Part model, mm, in its own coordinate system. A direction names the side the tool comes from. Give positions to 0.01 mm unless a question says otherwise; leave off trailing zeros. Order: outer loops, then holes, each group sorted by start corner. A loop starts at its lowest first (then second) coordinate and runs counter-clockwise, first axis right, second up.
1. Slice it at C-C on y = 4.2. List the corners of the cut face in (x, z).
2. Mould opens along X. For faces 1 (the flat face through (0, 2, -27)), 2 (the flat face through (31, 4, 0)), 3 (the cylindrical face through (32.287, 2.535, 26.248)) say: +X half, -X half, draft (parallel to the pull), parting line (faces both ways), or undercut.
3. Drop flat-ended pins along their axis: pin 1 Ø3 at (x, z) = (27, -22.5) entering from +Y; pin 2 Ø25 at (x, z) = (-1.5, 5.5) entering from +Y; pin 3 Ø3 at (x, z) = (-22, -16.5) entering from -Y. Give the stop position or say it passes through.
4. Slice it at B-B on x = -27. List the corners of the cut face in (y, z), and give its area (3 significant figures).
5. Slice it at D-D on z = 12. List the corners of the cut face in (x, y).
6. Slice it at A-A on z = -22. List the corners of the cut face in (x, y).
7. Probe line 1 (X direction, y = 1.1, z = -22); line 2 (Z direction, x = 27, y = 1.7); line 3 (X direction, y = 2.8, z = -22). List the from-to ranges inside material, lowest first.
8. Which spindle directions (+Z, -Z, +X, -X, +Y, -Y) get a long thin tool onto all of the face, cutting with end or side? Do faces 4 (the flat face through (0, 4, -25)), 5 (the cylindrical face through (-28.11, 1.52, -23.01)). Say none if no direction does.
from build123d import *

# Parameters (mm, degrees)
SKETCH1_W           = 66
SKETCH1_H           = 54
BOSS_EXTRUDE1_DEPTH = 5
SKETCH2_W           = 62
SKETCH2_H           = 50
CUT_EXTRUDE1_DEPTH  = 3
SKETCH3_W           = 8
SKETCH3_H           = 6
SKETCH3_R           = 1.5
BOSS_EXTRUDE2_DEPTH = 3
SKETCH4_R           = 1.5
CUT_EXTRUDE2_DEPTH  = 3
FILLET1_R           = 2.5


with BuildPart() as part:
    # Sketch1 → Boss-Extrude1 (new body)
    with BuildSketch(Plane(origin=(0, 0, 0), x_dir=(1, 0, 0), z_dir=(0, 1, 0))):
        Rectangle(SKETCH1_W, SKETCH1_H)
    extrude(amount=BOSS_EXTRUDE1_DEPTH)

    # Sketch2 → Cut-Extrude1 (cut)
    with BuildSketch(Plane(origin=(0, 5, 0), x_dir=(1, 0, 0), z_dir=(0, 1, 0))):
        Rectangle(SKETCH2_W, SKETCH2_H)
    extrude(amount=-CUT_EXTRUDE1_DEPTH, mode=Mode.SUBTRACT)

    # Sketch3 → Boss-Extrude2 (add)
    with BuildSketch(Plane(origin=(0, 0, 0), x_dir=(1, 0, 0), z_dir=(0, 1, 0))):
        with Locations((-27, -22)):
            Rectangle(SKETCH3_W, SKETCH3_H)
        with Locations((-27, -22)):
            Circle(SKETCH3_R, mode=Mode.SUBTRACT)
        with Locations((-27, 22)):
            Rectangle(SKETCH3_W, SKETCH3_H)
        with Locations((-27, 22)):
            Circle(SKETCH3_R, mode=Mode.SUBTRACT)
        with Locations((27, -22)):
            Rectangle(SKETCH3_W, SKETCH3_H)
        with Locations((27, -22)):
            Circle(SKETCH3_R, mode=Mode.SUBTRACT)
        with Locations((27, 22)):
            Rectangle(SKETCH3_W, SKETCH3_H)
        with Locations((27, 22)):
            Circle(SKETCH3_R, mode=Mode.SUBTRACT)
    extrude(amount=BOSS_EXTRUDE2_DEPTH)

    # Sketch4 → Cut-Extrude2 (cut)
    with BuildSketch(Plane(origin=(0, 2, 0), x_dir=(1, 0, 0), z_dir=(0, 1, 0))):
        with Locations((-27, 22)):
            Circle(SKETCH4_R)
        with Locations((-27, -22)):
            Circle(SKETCH4_R)
        with Locations((27, -22)):
            Circle(SKETCH4_R)
        with Locations((27, 22)):
            Circle(SKETCH4_R)
    extrude(amount=-CUT_EXTRUDE2_DEPTH, mode=Mode.SUBTRACT)

    # Fillet1
    fillet1_edges = [part.edges().sort_by_distance(p)[0] for p in [
        (33, 2.5, 27),
        (-33, 2.5, 27),
        (-33, 2.5, -27),
        (33, 2.5, -27),
    ]]
    fillet(fillet1_edges, radius=FILLET1_R)


solid = part.part
Data:
1. outline: (-33, -24.5) arc R2.5 ccw to (-30.5, -27) - (30.5, -27) arc R2.5 ccw to (33, -24.5) - (33, 24.5) arc R2.5 ccw to (30.5, 27) - (-30.5, 27) arc R2.5 ccw to (-33, 24.5) - close; hole (-31, -25) - (31, -25) - (31, 25) - (-31, 25) - close
2. face 1: draft
2. face 2: undercut
2. face 3: +X half
3. pin 1: stops at y = 3
3. pin 2: stops at y = 2
3. pin 3: stops at y = 0
4. outline: (0, -27) - (5, -27) - (5, -25) - (3, -25) - (3, -23.5) - (0, -23.5) - close; (0, -20.5) - (3, -20.5) - (3, -19) - (2, -19) - (2, 19) - (3, 19) - (3, 20.5) - (0, 20.5) - close; (0, 23.5) - (3, 23.5) - (3, 25) - (5, 25) - (5, 27) - (0, 27) - close
4. area: 114 mm2
5. outline: (-33, 0) - (33, 0) - (33, 5) - (31, 5) - (31, 2) - (-31, 2) - (-31, 5) - (-33, 5) - close
6. outline: (-33, 0) - (-28.5, 0) - (-28.5, 3) - (-31, 3) - (-31, 5) - (-33, 5) - close; (-25.5, 0) - (25.5, 0) - (25.5, 3) - (23, 3) - (23, 2) - (-23, 2) - (-23, 3) - (-25.5, 3) - close; (28.5, 0) - (33, 0) - (33, 5) - (31, 5) - (31, 3) - (28.5, 3) - close
7. line 1: x = -33 to -28.5, -25.5 to 25.5, 28.5 to 33
7. line 2: z = -27 to -23.5, -20.5 to 20.5, 23.5 to 27
7. line 3: x = -33 to -28.5, -25.5 to -23, 23 to 25.5, 28.5 to 33
8. face 4: +Y
8. face 5: +Y, -Y
